from build123d import *

# Parameters (mm, degrees)
SKETCH2_R          = 2.38125
CUT_EXTRUDE1_DEPTH = 9
CIRPATTERN1_COUNT  = 2
CIRPATTERN1_ANGLE  = 120


with BuildPart() as part:
    # Sketch1 → Revolve1 (revolve)
    with BuildSketch(Plane.XY):
        Polygon((4, 0), (-4, 0), (-4, 9.779), (-2.222, 9.779), (-2.222, 10.414), (2.222, 10.414), (2.222, 9.779), (4, 9.779), align=None)
    revolve(axis=Axis((8.430806561, 0, 0), (-1, 0, 0)))

    # Sketch2 → Cut-Extrude1 (cut, through all)
    with BuildSketch(Plane.ZY.offset(4)):
        Circle(SKETCH2_R)
    extrude(amount=-CUT_EXTRUDE1_DEPTH, mode=Mode.SUBTRACT)

    # Sketch4 → #8-32 Tapped Hole1 (revolve, cut)
    with BuildSketch(Plane(origin=(0, 10.414, 0), x_dir=(0, 0, 1), z_dir=(1, 0, 0))):
        Polygon((0, 0), (0, 13.483806461), (1.7272, 12.446), (1.7272, 0), align=None)
    f_8_32_tapped_hole1 = revolve(axis=Axis((0, 16.764, 0), (0, -1, 0)), mode=Mode.SUBTRACT)

    # CirPattern1: #8-32 Tapped Hole1 ×2 about axis
    cirpattern1_axis = Axis((4, 0, 0), (-1, 0, 0))
    for i in range(1, CIRPATTERN1_COUNT):
        add(f_8_32_tapped_hole1.rotate(cirpattern1_axis, i * CIRPATTERN1_ANGLE / (CIRPATTERN1_COUNT - 1)), mode=Mode.SUBTRACT)


solid = part.part
Can you work these out from the model? Positions are in its coordinate system, mm. A direction names the side the tool comes from. Give positions to 0.01 mm unless a question says otherwise; leave off trailing zeros. Loops run counter-clockwise (first coordinate to the right, second up) from the corner with the lowest first, then second, coordinate; pieces in that order, holes last. Notation, with made-up numbers: (-40, 25) - (11, 25) arc R24 cw to (11, 41) - close; hole circle Ø5 at (8.25, -4). An arc over 180 degrees is marked (long way). One line per item, written item: value.
(1) If we section it at C-C, the plane z = 6.25: List the corners of the cut face in (x, y) for me, plus the area to 3 significant figures.
Verdict:
outline: (-4, -7.52) - (-2.22, -7.52) - (-2.22, -8.33) - (2.22, -8.33) - (2.22, -7.52) - (4, -7.52) - (4, 7.52) - (2.22, 7.52) - (2.22, 8.33) - (-2.22, 8.33) - (-2.22, 7.52) - (-4, 7.52) - close
area: 128 mm^2
(2) If we section it at D-D, the plane y = -7.5: List the corners of the cut face in (x, z) for me.
Verdict:
outline: (-4, -6.28) - (-2.22, -6.28) - (-2.22, -7.23) - (2.22, -7.23) - (2.22, -6.28) - (4, -6.28) - (4, 6.28) - (2.22, 6.28) - (2.22, 7.23) - (-2.22, 7.23) - (-2.22, 6.28) - (-4, 6.28) - close
(3) I'm going to push flat-ended pins straight in: pin 1 (4 mm diameter, centred on x = 0, z = 0, fed in from +Y); pin 2 (3 mm diameter, centred on x = 1, z = 7, fed in from +Y); pin 3 (2 mm diameter, centred on x = 3, y = 1.5, fed in from +Z). Where does each tip first touch, or does it pass through?
Verdict:
pin 1: y = 10.41
pin 2: y = 8.84
pin 3: z = 10.38
(4) If we section it at A-A, the plane x = -2.5: List the corners of the cut face in (y, z) for me.
Verdict:
outline: circle Ø19.56 at (0, 0); hole circle Ø4.76 at (0, 0)
(5) If we section it at B-B, the plane y = 4.5: List the corners of the cut face in (x, z) for me, plus the area to 3 significant figures.
Verdict:
outline: (-4, -8.68) - (-2.22, -8.68) - (-2.22, -9.39) - (2.22, -9.39) - (2.22, -8.68) - (4, -8.68) - (4, 8.68) - (2.22, 8.68) - (2.22, 9.39) - (-2.22, 9.39) - (-2.22, 8.68) - (-4, 8.68) - close; hole circle Ø3.45 at (0, 0)
area: 136 mm^2
(6) On a 3-axis mill with a long thin cutter (end or side, diameter ignored), from which of +Z, -Z, +X, -X, +Y, -Y can I reach the whole of each face in a straight line? I mean faces 4 (the face through (-0.013, 1.185, 2.652)), 5 (the face through (-2.222, -8, 6)), 6 (the face through (2.222, 8, 6)). Say none if no direction works.
Verdict:
face 4: none
face 5: -X
face 6: +X
(7) If we mould it in two halves opening along Z, with no side actions, what happens to faces 1 (the face through (3.123, -2.12, 9.546)), 2 (the face through (-0.08, -4.54, -4.41)), 3 (the face through (-4, -2, 2))? For each: released by +Z, released by -Z, zero draft, split by the parting line, or undercut.
Verdict:
face 1: split by the parting line
face 2: undercut
face 3: zero draft
(8) I need wall thicknesses on line 1 along X through (y, z) = (5.75, 0); line 2 along Z through (x, y) = (-1.5, 0); line 3 along Z through (x, y) = (0, 4.25). Which ranges of each line are inside material? Lowest first, please.
Verdict:
line 1: -4 to -1.73, 1.73 to 4
line 2: -10.41 to -2.38, 2.38 to 10.41
line 3: -9.51 to -1.73, 1.73 to 9.51
